Geometry check sheet. Reference: the model listing, model coordinates, mm. A direction names the side the tool comes from. Give positions to 0.01 mm unless a question says otherwise; leave off trailing zeros. Loops run counter-clockwise (first coordinate to the right, second up) from the corner with the lowest first, then second, coordinate; pieces in that order, holes last. Notation, with made-up numbers: (55.5, -14) -> (107.5, -14) arc R12 ccw to (107.5, -6) -> close; hole circle Ø3 at (9, 35.25). An arc over 180 degrees is marked (long way). Write each question's results on one line, items separated by ' | '. Start each with the question number.
1) Depth check by flat-ended pin: pin 1 (1 mm diameter, centred on y = 0, z = -1.5, fed in from +X); pin 2 (1 mm diameter, centred on x = -1, y = 1.5, fed in from +Z); pin 3 (0.5 mm diameter, centred on x = 0.5, z = 1, fed in from -Y). Enter the tip coordinate at first touch or a pass-through.
2) Sectioned sample at A-A on z = -4.75. Record the cut outline in (x, y).
3) Draft check along X on faces 1 (the face through (0, 2, 0)), 2 (the face through (-1.5, 0.07, -4.84)), 3 (the face through (0, 1, 1)). Enter one of: pulls with the +X half, pulls with the -X half, needs draft (parallel to the pull), parting line crosses it, or undercut.
4) Set-up check for faces 4 (the face through (0.87, -0.49, 1.06)), 5 (the face through (0, 0, -10)): record each of +Z, -Z, +X, -X, +Y, -Y from which the full face is reachable in a straight line by a thin tool's end or side.
5) Scan lines: line 1 (Y direction, x = 0, z = -5.75); line 2 (Z direction, x = 0.35, y = 1.8). Record each from-to range of solid material in increasing order. Write a range as from..to.
Solid Edge part; units mm, degrees
sketch "Sketch1" plane through (0, 0, 0) normal (0, -1, 0) x (1, 0, 0)
  line L0 (0, -10) -> (1.5, -10)
  line L1 (1.5, -10) -> (1.5, -0.115)
  arc A0 (1.5, -0.105) -> (1.5, -0.115) centre (1.5038, -0.11) ccw
  line L2 (1.5, -0.105) -> (1.5, 0)
  line L3 (1.5, 0) -> (2.85, 0)
  line L4 (2.85, 0) -> (2.85, 0.165)
  arc A1 (1.27, 1.65) -> (2.85, 0.165) centre (-0.3628, -1.6703) cw
  line L5 (0, 1.65) -> (1.27, 1.65)
  dimension "D1" = 1.5
revolve "RevolvedProtrusion1" add sketch "Sketch1" angle 360 about axis through (0, 0, 5) along (0, 0, -1)
sketch "Sketch2" plane through (0, 0, 0) normal (0, -1, 0) x (1, 0, 0)
  line L0 (0, -0.0566) -> (1.1545, 0.61)
  line L1 (1.1545, 0.61) -> (1.1545, 1.65)
  line L2 (1.1545, 1.65) -> (0, 1.65)
revolve "RevolvedCutout1" cut sketch "Sketch2" angle 360 about axis through (0, 0, 5.3) along (0, 0, -1)
sketch "Sketch3" plane through (0, 0, 0) normal (0, 0, -1) x (0, 1, 0)
  arc A0 (-1, 0.577) -> (-1, -0.577) centre (0, 0) ccw
  line L0 (-1, 0.577) -> (-1, -0.577)
extrude "Protrusion1" add sketch "Sketch3" against normal blind 1.65
pattern_circular "Pattern1" count 6 over 360 about axis through (0, 0, 0) along (0, 0, -1) of "Protrusion1"
fillet "Round_1" radius 0.185 1 edges at (-1.27, 0, 1.65)
sketch "Sketch4" plane through (0, 0, 0) normal (0, -1, 0) x (1, 0, 0)
  line L0 (0, 0.9501) -> (1.2122, 1.65)
  line L1 (1.2122, 1.65) -> (0, 1.65)
revolve "RevolvedCutout2" cut sketch "Sketch4" angle 360 about axis through (0, 0, 5.3) along (0, 0, -1)
sketch "Sketch5" plane through (0, 0, 0) normal (0, -1, 0) x (1, 0, 0)
  line L0 (-1.5, 0) -> (-1.5, -0.1)
  line L1 (-1.6, 0) -> (-1.5, 0)
  arc A0 (-1.6, 0) -> (-1.5, -0.1) centre (-1.6, -0.1) cw
revolve "RevolvedProtrusion2" add sketch "Sketch5" angle 360 about axis through (0, 0, -0.5) along (0, 0, 1)
cosmetic_thread "Thread1"
chamfer "Chamfer1" distance 0.3065 angle 45 1 edges at (-1.5, 0, -10)
properties material "Stahl"
Result:
1) pin 1: x = 1.5 | pin 2: z = 1.63 | pin 3: y = -2.39
2) outline: circle Ø3 at (0, 0)
3) face 1: needs draft | face 2: parting line crosses it | face 3: undercut
4) face 4: +Z | face 5: -Z, +X, -X, +Y, -Y
5) line 1: -1.5..1.5 | line 2: 0..1.31
